Geometry: see drawing. Coordinates: mm, zero at the bounding-box minimum. A direction names the side the tool comes from. Give positions to 0.01 mm unless a question says otherwise; leave off trailing zeros. Write each loop counter-clockwise with the first axis right and the second up, starting at its lowest first coordinate (ties: lowest second). Pieces come first, ordered by that corner, then holes. Notation, with made-up numbers: (75.25, 64) - (117.25, 64) arc R28 ccw to (117.25, 92) - close; hole circle Ø6 at (48, -27.75). An arc over 180 degrees is marked (long way). Use a Markdown table: item, result. Add a question column.
1. Material intervals for probe 1 along Y at (x, z) = (11.25, 25.25) (1 decimal); probe 2 along Z at (x, y) = (18.5, 9.25); probe 3 along Y at (x, z) = (1, 17.5) (1 decimal), sorted ascending.
2. Section query D-D, the plane z = 10.5. Return loops of the section in (x, y) (1 decimal).
3. Section query B-B, the plane y = 5.75. Return loops of the section in (x, z).
4. Mould query, pull axis Y, two halves, no side actions, for the marked faces 4, 5, 6 and 7. Classes: released by +Y, released by -Y, zero draft, split by the parting line, or undercut.
5. Pin query (flat end, axial travel): pin 1 (0.8 mm diameter, centred on y = 16, z = 13.5, fed in from -X); pin 2 (2 mm diameter, centred on x = 15.5, y = 4, fed in from -Z); pin 3 (6.5 mm diameter, centred on x = 11, z = 12.5, fed in from +Y); pin 4 (3 mm diameter, centred on x = 1.5, z = 14, fed in from +Y). Return the tip coordinate at first contact, or that it passes through.
6. Section query C-C, the plane x = 8. Return loops of the section in (y, z) (1 decimal), plus the area to 3 significant figures.
7. Section query A-A, the plane z = 14. Return loops of the section in (x, y) (1 decimal), plus the area to 3 significant figures.
8. Set-up query: the marked faces 1, 2 and 3. Return all of +Z, -Z, +X, -X, +Y, -Y with unobstructed straight access to the full face (end or side cutting, diameter ignored); none if empty.
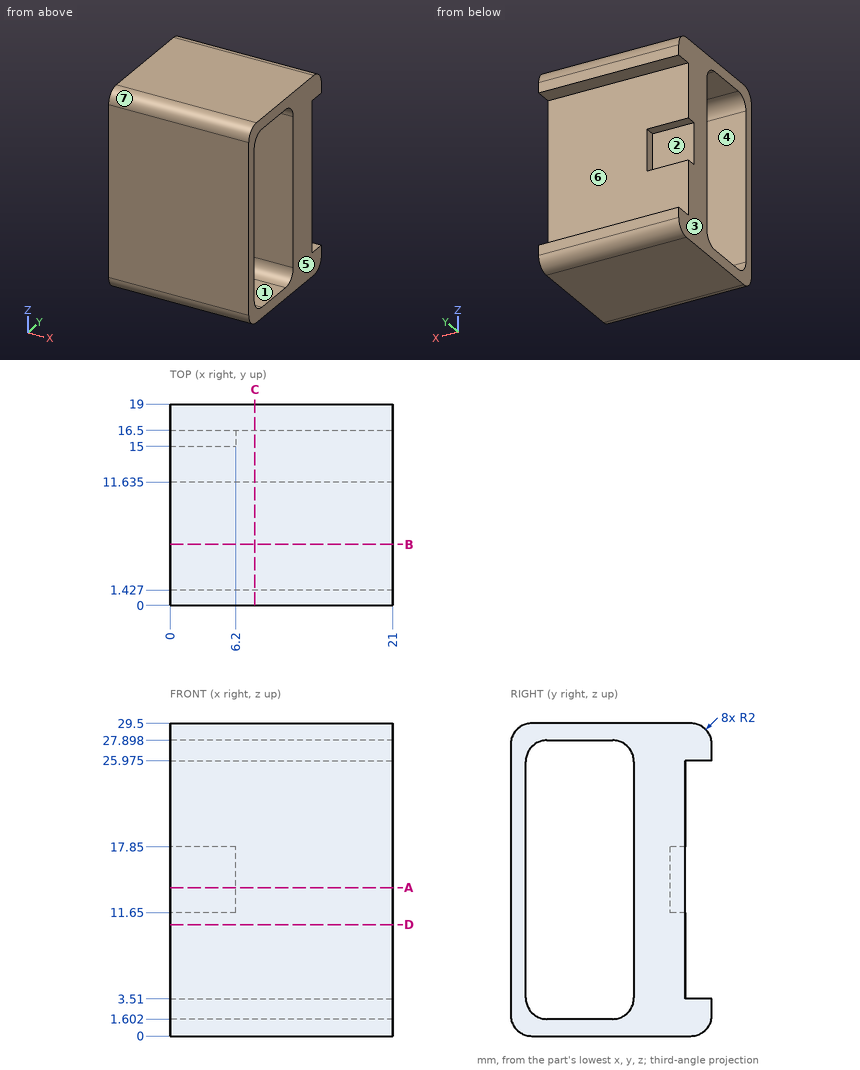
Result sheet:
| question | item | result |
|---|---|---|
| 1 | probe 1 | y = 0 to 1.4, 11.6 to 16.5 |
| 1 | probe 2 | z = 0 to 1.6, 27.9 to 29.5 |
| 1 | probe 3 | y = 0 to 1.4, 11.6 to 15 |
| 2 | outline | (0, 0) - (21, 0) - (21, 1.4) - (0, 1.4) - close; (0, 11.6) - (21, 11.6) - (21, 16.5) - (0, 16.5) - close |
| 3 | outline | (0, 0) - (21, 0) - (21, 1.6) - (0, 1.6) - close; (0, 27.9) - (21, 27.9) - (21, 29.5) - (0, 29.5) - close |
| 4 | face 4 | undercut |
| 4 | face 5 | zero draft |
| 4 | face 6 | released by +Y |
| 4 | face 7 | released by -Y |
| 5 | pin 1 | stops at x = 6.2 |
| 5 | pin 2 | stops at z = 0 |
| 5 | pin 3 | stops at y = 16.5 |
| 5 | pin 4 | stops at y = 15 |
| 6 | outline | (0, 2) arc R2 ccw to (2, 0) - (17, 0) arc R2 ccw to (19, 2) - (19, 3.5) - (16.5, 3.5) - (16.5, 26) - (19, 26) - (19, 27.5) arc R2 ccw to (17, 29.5) - (2, 29.5) arc R2 ccw to (0, 27.5) - close; hole (1.4, 3.6) arc R2 ccw to (3.4, 1.6) - (9.6, 1.6) arc R2 ccw to (11.6, 3.6) - (11.6, 25.9) arc R2 ccw to (9.6, 27.9) - (3.4, 27.9) arc R2 ccw to (1.4, 25.9) - close |
| 6 | area | 236 mm² |
| 7 | outline | (0, 0) - (21, 0) - (21, 1.4) - (0, 1.4) - close; (0, 11.6) - (21, 11.6) - (21, 16.5) - (6.2, 16.5) - (6.2, 15) - (0, 15) - close |
| 7 | area | 123 mm² |
| 8 | face 1 | +X, -X |
| 8 | face 2 | -X, +Y |
| 8 | face 3 | +Z, -Z, -X, +Y, -Y |
